```python
from build123d import *

# Parameters (mm, degrees)
F0_W     = 70.7396790385
F0_H     = 59.6152953804
F1_DEPTH = 25.4
F2_R     = 16.4409735045
F3_DEPTH = 25.4
F5_D     = 6.35


with BuildPart() as f1:
    # F0 (on Front) → F1 (new body)
    with BuildSketch(Plane.XZ):
        Polygon((0, 56.6202700138), (-35.3698395193, 29.8076476902), (35.3698395193, 29.8076476902), align=None)
        Rectangle(F0_W, F0_H)
        Polygon((-35.3698395193, -29.8076476902), (-35.3698395193, 29.8076476902), (-62.7529397607, 0), align=None)
        Polygon((59.6152916551, 0), (35.3698395193, 29.8076476902), (35.3698395193, -29.8076476902), align=None)
        Polygon((35.3698395193, -29.8076476902), (-35.3698395193, -29.8076476902), (0, -56.3350282609), align=None)
    extrude(amount=F1_DEPTH)

    # F2 (on Front) → F3 (join)
    with BuildSketch(Plane.XZ):
        Circle(F2_R)
    extrude(amount=F3_DEPTH)

    # F5 (through all)
    with Locations(Plane(origin=(0, 0, 0), x_dir=(1, 0, 0), z_dir=(0, 1, 0))):
        with Locations((0, -22.0009903873)):
            Hole(F5_D / 2)


solid = f1.part
```
Geometry: final body of the model. Coordinates: model frame, mm. Round coordinates to 2 decimals unless told otherwise and drop trailing zeros. Write each loop counter-clockwise with the first axis right and the second up, starting at its lowest first coordinate (ties: lowest second). Pieces come first, ordered by that corner, then holes. Notation, with made-up numbers: (73, 3) -> (120, 3) arc R18 cw to (120, 34) -> close; hole circle Ø6 at (74.25, -4.5). An arc over 180 degrees is marked (long way). Return JSON: item names as keys, results as strings.
Q1. Ray query, line 1 (Z direction, x = 0, y = -17); line 2 (X direction, y = -10, z = 22.5); line 3 (X direction, y = -8.25, z = 52.5). Return the intervals inside material, ascending.
From the geometry:
{"line 1": "-56.34 to 18.83, 25.18 to 56.62", "line 2": "-42.08 to -3.14, 3.14 to 41.31", "line 3": "-5.44 to 5.44"}
Q2. Section A-A on y = -12. Return the cut outline in (x, z) (3 decimals).
From the geometry:
{"outline": "(-62.753, 0) -> (-35.37, -29.808) -> (0, -56.335) -> (35.37, -29.808) -> (59.615, 0) -> (35.37, 29.808) -> (0, 56.62) -> (-35.37, 29.808) -> close; hole circle Ø6.35 at (0, 22.001)"}
Q3. Section B-B on z = -38. Return the cut outline in (x, y).
From the geometry:
{"outline": "(-24.45, -25.4) -> (24.45, -25.4) -> (24.45, 0) -> (-24.45, 0) -> close"}
Q4. Section C-C on x = 32. Return the cut outline in (y, z).
From the geometry:
{"outline": "(-25.4, -32.34) -> (0, -32.34) -> (0, 32.36) -> (-25.4, 32.36) -> close"}
Q5. Mould query, pull axis Z, two halves, no side actions, for faces 1 (the cylindrical face through (0.413, -12.878, 18.853)), 2 (the flat face through (-48.87, -12.52, 15.11)), 3 (the flat face through (17.437, -12.522, -43.257)), 4 (the flat face through (-2, 0, 1)). Classes: +Z half, -Z half, draft (parallel to the pull), parting line (faces both ways), or undercut.
From the geometry:
{"face 1": "undercut", "face 2": "+Z half", "face 3": "-Z half", "face 4": "draft"}
Q6. First-contact query: pin 1 Ø2 at (x, y) = (42.5, -4.5) entering from +Z; pin 2 Ø8 at (y, z) = (-13, 23.5) entering from -X; pin 3 Ø2 at (x, y) = (-35.5, -13.5) entering from -Z. Flat tips, straight axial feed; report the tip coordinate or a pass-through.
From the geometry:
{"pin 1": "z = 22.27", "pin 2": "x = -44.84", "pin 3": "z = -30.46"}
